Input: part model. Units: mm. Frame: model coordinates. Face numbers are marked on the shaded views. Coordinates: 2 decimals unless noted, no trailing zeros. Order: outer loops, then holes, each group sorted by start corner. A loop starts at its lowest first (then second) coordinate and runs counter-clockwise, first axis right, second up. Notation, with made-up numbers: (31, 89) -> (45, 89) arc R18 cw to (45, 123) -> close; hole circle Ø6 at (34.5, 69.5). An arc over 180 degrees is marked (long way). One line per question, with ' | ' between items.
```python
from build123d import *

# Parameters (mm, degrees)
ESTRUSIONE_ESTRUSIONE1_DEPTH      = 48
ESTRUSIONE_ESTRUSIONE1_DEPTH_BACK = 5
SCHIZZO1_W                        = 79.084596206
SCHIZZO1_H                        = 3
SCHIZZO2_W                        = 45
SCHIZZO2_H                        = 3
ESTRUSIONE_ESTRUSIONE2_DEPTH      = 5
SCHIZZO3_W                        = 60
SCHIZZO3_H                        = 37
TAGLIO_ESTRUSIONE1_DEPTH          = 10
SCHIZZO4_W                        = 20
SCHIZZO4_H                        = 8
ESTRUSIONE_ESTRUSIONE3_DEPTH      = 3


with BuildPart() as part:
    # Schizzo1 → Estrusione-Estrusione1 (new, two sides: drawn at the far end of the back side and taken through both)
    with BuildSketch(Plane.XY.offset(-ESTRUSIONE_ESTRUSIONE1_DEPTH_BACK)):
        with Locations((119.542298103, -82.5)):
            Rectangle(SCHIZZO1_W, SCHIZZO1_H)
    extrude(amount=ESTRUSIONE_ESTRUSIONE1_DEPTH + ESTRUSIONE_ESTRUSIONE1_DEPTH_BACK)

    # Schizzo2 → Estrusione-Estrusione2 (add)
    with BuildSketch(Plane(origin=(159.084596206, 0, 0), x_dir=(0, 0, -1), z_dir=(1, 0, 0))):
        with Locations((-22.5, -82.5)):
            Rectangle(SCHIZZO2_W, SCHIZZO2_H)
    estrusione_estrusione2 = extrude(amount=ESTRUSIONE_ESTRUSIONE2_DEPTH)

    # Specchia1: Estrusione-Estrusione2 across plane
    add(estrusione_estrusione2.mirror(Plane(origin=(119.542298103, 0, 0), x_dir=(0, 0, 1), z_dir=(1, 0, 0))))

    # Schizzo3 → Taglio-Estrusione1 (cut)
    with BuildSketch(Plane(origin=(0, -81, 0), x_dir=(1, 0, 0), z_dir=(0, 1, 0))):
        with Locations((105, -22.5)):
            Rectangle(SCHIZZO3_W, SCHIZZO3_H)
    extrude(amount=-TAGLIO_ESTRUSIONE1_DEPTH, mode=Mode.SUBTRACT)

    # Schizzo4 → Estrusione-Estrusione3 (add)
    with BuildSketch(Plane.XZ.offset(81)):
        with Locations((105, 41)):
            Rectangle(SCHIZZO4_W, SCHIZZO4_H)
    extrude(amount=-ESTRUSIONE_ESTRUSIONE3_DEPTH)


solid = part.part
```
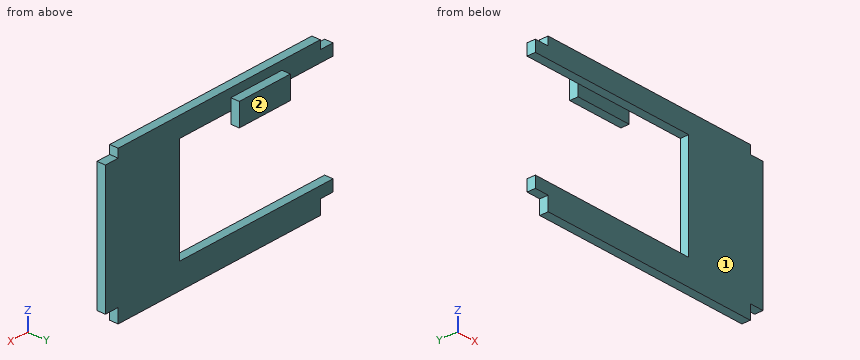
1. Cut plane C-C, the plane z = 26.5. Return loops of the section in (x, y).
Recorded:
outline: (135, -84) -> (164.08, -84) -> (164.08, -81) -> (135, -81) -> close
2. Cut plane B-B, the plane y = -82.35. Return loops of the section in (x, z).
Recorded:
outline: (75, 0) -> (80, 0) -> (80, -5) -> (159.08, -5) -> (159.08, 0) -> (164.08, 0) -> (164.08, 45) -> (159.08, 45) -> (159.08, 48) -> (80, 48) -> (80, 45) -> (75, 45) -> (75, 41) -> (135, 41) -> (135, 4) -> (75, 4) -> close
3. Mould query, pull axis Y, two halves, no side actions, for the marked faces 1 and 2. Classes: released by +Y, released by -Y, zero draft, split by the parting line, or undercut.
Recorded:
face 1: released by -Y | face 2: released by +Y
4. Cut plane A-A, the plane x = 116. Return loops of the section in (y, z).
Recorded:
outline: (-84, -5) -> (-81, -5) -> (-81, 4) -> (-84, 4) -> close; (-84, 41) -> (-81, 41) -> (-81, 48) -> (-84, 48) -> close
5. Cut plane D-D, the plane x = 146. Return loops of the section in (y, z).
Recorded:
outline: (-84, -5) -> (-81, -5) -> (-81, 48) -> (-84, 48) -> close
6. Pin query (flat end, axial travel): pin 1 Ø2.5 at (x, y) = (77, -83) entering from +Z; pin 2 Ø1.5 at (y, z) = (-82.5, -1.5) entering from -X; pin 3 Ø1.5 at (y, z) = (-82, 14.5) entering from -X. Return the tip coordinate at first contact, or that it passes through.
Recorded:
pin 1: stops at z = 45 | pin 2: stops at x = 80 | pin 3: stops at x = 135
7. Ray query, line 1 (Z direction, x = 93.5, y = -83.6); line 2 (X direction, y = -83.4, z = 23.5); line 3 (Z direction, x = 105, y = -80.3). Return the intervals inside material, ascending. Write a range as [from, to].
Recorded:
line 1: z = [-5, 4], [41, 48] | line 2: x = [135, 164.08] | line 3: z = [37, 45]
